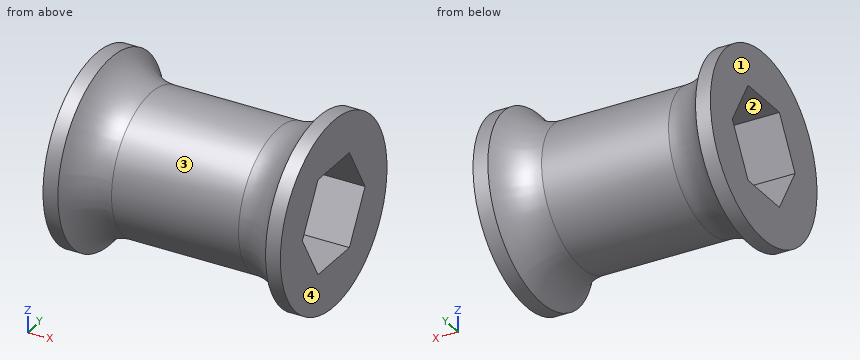
from build123d import *

# Parameters (mm, degrees)
CUT_EXTRUDE1_DEPTH = 33.385


with BuildPart() as part:
    # Sketch1 → Revolve1 (revolve)
    with BuildSketch(Plane.XY):
        with BuildLine():
            Line((0, 0), (0, 12.7))
            Line((0, 12.7), (2.032, 12.7))
            ThreePointArc((2.032, 12.7), (4.356261314, 10.375738686), (7.531261314, 9.525))
            Line((7.531261314, 9.525), (24.853738686, 9.525))
            ThreePointArc((24.853738686, 9.525), (28.028738686, 10.375738686), (30.353, 12.7))
            Line((30.353, 12.7), (32.385, 12.7))
            Line((32.385, 12.7), (32.385, 0))
            Line((32.385, 0), (0, 0))
        make_face()
    revolve(axis=Axis((0, 0, 0), (-1, 0, 0)))

    # Sketch2 → Cut-Extrude1 (cut, through all)
    with BuildSketch(Plane.ZY):
        Polygon((0, 7.478995387), (-6.477, 3.739497694), (-6.477, -3.739497694), (0, -7.478995387), (6.477, -3.739497694), (6.477, 3.739497694), align=None)
    extrude(amount=-CUT_EXTRUDE1_DEPTH, mode=Mode.SUBTRACT)


solid = part.part
Source: CAD feature listing. Evaluate the final solid. Frame: model axes, mm. Face numbers are marked on the shaded views. Round coordinates to 2 decimals unless told otherwise and drop trailing zeros. Loops run counter-clockwise (first coordinate to the right, second up) from the corner with the lowest first, then second, coordinate; pieces in that order, holes last. Notation, with made-up numbers: (28, 2) - (77, 2) arc R31 ccw to (77, 30) - close; hole circle Ø5 at (15.25, 62). An arc over 180 degrees is marked (long way). Write item = value, one per line. Start each with the question number.
(1) Pull-direction query (X, two-part tool) for the marked faces 1, 2, 3 and 4; classes: +X half, -X half, draft (parallel to the pull), parting line (faces both ways), or undercut.
(2) Pin query (flat end, axial travel): pin 1 (8 mm diameter, centred on x = 8.5, y = 1, fed in from -Z); pin 2 (6 mm diameter, centred on x = 16.5, y = -2.5, fed in from -Z) (3 decimals); pin 3 (10 mm diameter, centred on y = -8, z = -6, fed in from -X); pin 4 (1 mm diameter, centred on x = 6, y = -1.5, fed in from +Z). Return the tip coordinate at first contact, or that it passes through.
(3) Section query C-C, the plane x = 4. Output: boundary loops of the cut face in (y, z).
(4) Section query A-A, the plane y = 0. Output: boundary loops of the cut face in (x, z) (3 decimals).
(5) Ray query, line 1 along Z through (x, y) = (24.5, 0) (3 decimals); line 2 along Z through (x, y) = (23, -6.5); line 3 along Y through (x, z) = (13, -5). Return the intervals inside material, ascending. Write a range as from..to.
Conclusion:
q1.face_1 = -X half
q1.face_2 = draft
q1.face_3 = undercut
q1.face_4 = +X half
q2.pin_1 = -10.27
q2.pin_2 = -9.525
q2.pin_3 = 0
q2.pin_4 = 9.76
q3.outline = circle Ø21.19 at (0, 0); hole (-7.48, 0) - (-3.74, -6.48) - (3.74, -6.48) - (7.48, 0) - (3.74, 6.48) - (-3.74, 6.48) - close
q4.outline = (0, -12.7) - (2.032, -12.7) arc R6.35 cw to (7.531, -9.525) - (24.854, -9.525) arc R6.35 cw to (30.353, -12.7) - (32.385, -12.7) - (32.385, -6.477) - (0, -6.477) - close; (0, 6.477) - (32.385, 6.477) - (32.385, 12.7) - (30.353, 12.7) arc R6.35 cw to (24.854, 9.525) - (7.531, 9.525) arc R6.35 cw to (2.032, 12.7) - (0, 12.7) - close
q5.line_1 = -9.525..-6.477, 6.477..9.525
q5.line_2 = -6.96..-1.7, 1.7..6.96
q5.line_3 = -8.11..-4.59, 4.59..8.11
